Autodesk Inventor part; units mm, degrees
ref_plane "Plano inicial" through (0, 0, 0) normal (0, 0, 1) x (1, 0, 0)
ref_plane "Plano final" through (0, 0, 1700) normal (0, 0, 1) x (1, 0, 0)
ref_plane "YZ Plane" through (0, 0, 0) normal (1, 0, 0) x (0, 1, 0)
ref_plane "Plano inicial" through (0, 0, 0) normal (0, 0, 1) x (1, 0, 0)
ref_plane "Plano final" through (0, 0, 1700) normal (0, 0, 1) x (1, 0, 0)
sketch "Boceto" plane through (0, 0, 0) normal (0, 0, 1) x (1, 0, 0)
  line L0 (-25.4, -19.05) -> (-25.4, 19.05)
  line L1 (-19.05, 25.4) -> (19.05, 25.4)
  line L2 (25.4, 19.05) -> (25.4, -19.05)
  line L3 (19.05, -25.4) -> (-19.05, -25.4)
  arc A0 (-25.4, -19.05) -> (-19.05, -25.4) centre (-19.05, -19.05) ccw
  arc A1 (-19.05, 25.4) -> (-25.4, 19.05) centre (-19.05, 19.05) ccw
  arc A2 (25.4, 19.05) -> (19.05, 25.4) centre (19.05, 19.05) ccw
  arc A3 (19.05, -25.4) -> (25.4, -19.05) centre (19.05, -19.05) ccw
  arc A4 (-19.05, 22.225) -> (-22.225, 19.05) centre (-19.05, 19.05) ccw
  line L4 (-19.05, 22.225) -> (19.05, 22.225)
  arc A5 (22.225, 19.05) -> (19.05, 22.225) centre (19.05, 19.05) ccw
  line L5 (22.225, 19.05) -> (22.225, -19.05)
  arc A6 (19.05, -22.225) -> (22.225, -19.05) centre (19.05, -19.05) ccw
  line L6 (19.05, -22.225) -> (-19.05, -22.225)
  arc A7 (-22.225, -19.05) -> (-19.05, -22.225) centre (-19.05, -19.05) ccw
  line L7 (-22.225, -19.05) -> (-22.225, 19.05)
  line L8 (0, 37.4012) -> (0, -37.4012) construction
  line L9 (-37.4012, 0) -> (37.4012, 0) construction
  dimension "d10" = 50.8
  dimension "d11" = 50.8
  dimension "d12" = 3.175
  dimension "d15" = 25.4
  dimension "d16" = 25.4
  dimension "d17" = 6.35
extrude "Cuerpo" add sketch "Boceto" along normal up to surface (1700 mm away) from surface at 0
sketch "Sketch3" plane through (0, 0, 0) normal (0, 0, 1) x (1, 0, 0)
  line L0 (0, 0) -> (10, 0)
ref_plane "Work Plane3" through (0, 0, 0) normal (0, -1, 0) x (1, 0, 0)
sketch "Sketch4" plane through (0, 0, 0) normal (0, -1, 0) x (1, 0, 0)
  line L0 (-2, 0) -> (12, 0)
  line L1 (-2, 1700) -> (12, 1700)
  dimension "d19" = 1700
equation "\"d10\" = G_H"
equation "\"d11\" = G_W"
equation "\"d12\" = G_T"
equation "\"d15\" = 0.5 * d10"
equation "\"d16\" = 0.5 * d11"
equation "\"d17\" = G_IR"
equation "\"d3\" = G_L"
equation "\"G_W\" = 50.8"
equation "\"G_H\" = 50.8"
equation "\"G_T\" = 3.175"
equation "\"G_IR\" = 6.35"
equation "\"G_L\" = d19"
equation "\"G_OFFSET_START\" = 0"
equation "\"G_OFFSET_END\" = 0"
equation "\"d14\" = G_OFFSET_END + B_L"
equation "\"B_L\" = 1700"
properties part number "AISC - 2 x 2 x 1/8 - 66,929" material "Acero, suave"
Source: CAD feature listing. Evaluate the final solid. Frame: model axes, mm. A direction names the side the tool comes from. Coordinates: 2 decimals unless noted, no trailing zeros. Loops run counter-clockwise (first coordinate to the right, second up) from the corner with the lowest first, then second, coordinate; pieces in that order, holes last. Notation, with made-up numbers: (64.25, 86) - (75.25, 86) arc R31 cw to (75.25, 117) - close; hole circle Ø4 at (-0.75, 24). An arc over 180 degrees is marked (long way). One line per item, written item: value. Start each with the question number.
1. Section C-C (z = 959). Return the cut outline in (x, y) (3 decimals), and give its area (3 significant figures).
2. Contact query for a flat-ended pin moving along its axis: P1, Ø12, axis at x = -1.5, y = 20, coming from the +Z side. Output: stop coordinate, or through.
3. Section A-A (x = 9). Return the cut outline in (y, z) (3 decimals), and give its area (3 significant figures).
4. Ray query, L1, parallel to Y at x = 16, z = 358.5 (3 decimals); L2, parallel to X at y = -21.5, z = 1185. Return the intervals inside material, ascending.
5. Set-up query: faces 1 (the flat face through (0, 22.225, 838)), 2 (the flat face through (-25.4, 0, 838)). Return all of +Z, -Z, +X, -X, +Y, -Y with unobstructed straight access to the full face (end or side cutting, diameter ignored); none if empty.
6. Mould query, pull axis Y, two halves, no side actions, for faces 3 (the flat face through (22.225, 0, 838)), 4 (the flat face through (0, -25.4, 838)), 5 (the flat face through (-0.1, -22.5, 0)). Classes: pulls with the +Y half, pulls with the -Y half, needs draft (parallel to the pull), parting line crosses it, or undercut.
Verdict:
1. outline: (-25.4, -19.05) arc R6.35 ccw to (-19.05, -25.4) - (19.05, -25.4) arc R6.35 ccw to (25.4, -19.05) - (25.4, 19.05) arc R6.35 ccw to (19.05, 25.4) - (-19.05, 25.4) arc R6.35 ccw to (-25.4, 19.05) - close; hole (-22.225, -19.05) arc R3.175 ccw to (-19.05, -22.225) - (19.05, -22.225) arc R3.175 ccw to (22.225, -19.05) - (22.225, 19.05) arc R3.175 ccw to (19.05, 22.225) - (-19.05, 22.225) arc R3.175 ccw to (-22.225, 19.05) - close
1. area: 579 mm2
2. P1: stops at z = 1700
3. outline: (-25.4, 0) - (-22.225, 0) - (-22.225, 1700) - (-25.4, 1700) - close; (22.225, 0) - (25.4, 0) - (25.4, 1700) - (22.225, 1700) - close
3. area: 10,800 mm2
4. L1: y = -25.4 to -22.225, 22.225 to 25.4
4. L2: x = -24.91 to -21.07, 21.07 to 24.91
5. face 1: +Z, -Z
5. face 2: +Z, -Z, -X, +Y, -Y
6. face 3: undercut
6. face 4: pulls with the -Y half
6. face 5: needs draft
